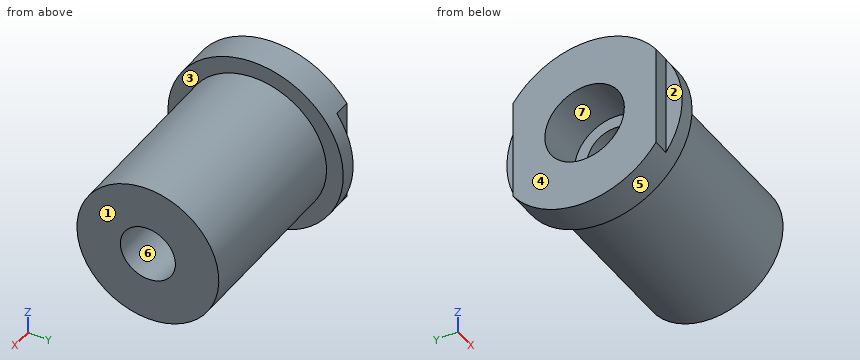
from build123d import *

# Parameters (mm, degrees)
ESQUISSE2_W                  = 103
ESQUISSE2_H                  = 43
ESQUISSE3_OUTSIDE_W          = 119.876
ESQUISSE3_OUTSIDE_H          = 119.876
ESQUISSE3_OUTSIDE_R          = 34.8
ENL_V_MAT_EXTRU_1_DEPTH      = 87
ENL_V_MAT_EXTRU_2_DEPTH      = 120.61187232
ENL_V_MAT_EXTRU_2_DEPTH_BACK = 8
ENL_V_MAT_EXTRU_3_DEPTH      = 120.61187232
ENL_V_MAT_EXTRU_3_DEPTH_BACK = 8
ESQUISSE7_R                  = 19.5
ENL_V_MAT_EXTRU_4_DEPTH      = 24
ESQUISSE8_R                  = 13.5
ENL_V_MAT_EXTRU_5_DEPTH      = 100.694533451


with BuildPart() as part:
    # Esquisse2 → Révolution1 (revolve)
    with BuildSketch(Plane.XY, mode=Mode.PRIVATE) as r_volution1_sk:
        with Locations((51.5, 21.5)):
            Rectangle(ESQUISSE2_W, ESQUISSE2_H)
    revolve(r_volution1_sk.sketch.rotate(Axis((103, 0, 0), (-1, 0, 0)), 90), axis=Axis((103, 0, 0), (-1, 0, 0)))

    # Esquisse3 outside → Enlèv. mat.-Extru.1 (cut)
    with BuildSketch(Plane(origin=(103, 0, 0), x_dir=(0, 0, -1), z_dir=(1, 0, 0))):
        Rectangle(ESQUISSE3_OUTSIDE_W, ESQUISSE3_OUTSIDE_H)
        Circle(ESQUISSE3_OUTSIDE_R, mode=Mode.SUBTRACT)
    extrude(amount=-ENL_V_MAT_EXTRU_1_DEPTH, mode=Mode.SUBTRACT)

    # Esquisse4 → Enlèv. mat.-Extru.2 (cut, two sides: drawn at the far end of the back side and taken through both)
    with BuildSketch(Plane.ZY.offset(-ENL_V_MAT_EXTRU_2_DEPTH_BACK)):
        Polygon((-241.912631386, 35), (-24.979991994, 35), (24.979991994, 35), (241.912631386, 35), (241.912631386, 468.865278784), (-241.912631386, 468.865278784), align=None)
    extrude(amount=ENL_V_MAT_EXTRU_2_DEPTH + ENL_V_MAT_EXTRU_2_DEPTH_BACK, mode=Mode.SUBTRACT)

    # Esquisse5 → Enlèv. mat.-Extru.3 (cut, two sides: drawn at the far end of the back side and taken through both)
    with BuildSketch(Plane.ZY.offset(-ENL_V_MAT_EXTRU_3_DEPTH_BACK)):
        Polygon((-241.912631386, -35), (-24.979991994, -35), (24.979991994, -35), (241.912631386, -35), (241.912631386, -468.865278784), (-241.912631386, -468.865278784), align=None)
    extrude(amount=ENL_V_MAT_EXTRU_3_DEPTH + ENL_V_MAT_EXTRU_3_DEPTH_BACK, mode=Mode.SUBTRACT)

    # Esquisse7 → Enlèv. mat.-Extru.4 (cut)
    with BuildSketch(Plane.ZY):
        Circle(ESQUISSE7_R)
    extrude(amount=-ENL_V_MAT_EXTRU_4_DEPTH, mode=Mode.SUBTRACT)

    # Esquisse8 → Enlèv. mat.-Extru.5 (cut, through all)
    with BuildSketch(Plane.ZY.offset(-24)):
        Circle(ESQUISSE8_R)
    extrude(amount=-ENL_V_MAT_EXTRU_5_DEPTH, mode=Mode.SUBTRACT)


solid = part.part
Input: part model. Units: mm. Frame: model coordinates. Face numbers are marked on the shaded views. A direction names the side the tool comes from. Coordinates: 2 decimals unless noted, no trailing zeros. Loops run counter-clockwise (first coordinate to the right, second up) from the corner with the lowest first, then second, coordinate; pieces in that order, holes last.
Q1. Cut plane A-A (y = 0). Output: boundary loops of the cut face in (x, z).
Q2. Contact query for flat-ended pins moving along their axis: pin 1 (6.5 mm diameter, centred on x = 2.5, z = 3.5, fed in from -Y); pin 2 (3 mm diameter, centred on x = 41, y = -15.5, fed in from -Z); pin 3 (5 mm diameter, centred on x = 14.5, z = -3, fed in from -Y); pin 4 (16 mm diameter, centred on y = 0, z = 0, fed in from -X). Output: stop coordinate, or through.
Q3. Draft query along Y for the marked faces 4, 5, 6 and 7. Return one class per face: +Y half, -Y half, draft (parallel to the pull), parting line (faces both ways), or undercut.
Q4. Material intervals for line 1 (Y direction, x = 5.5, z = 0); line 2 (Y direction, x = 11.25, z = 0); line 3 (X direction, y = 23.5, z = 27), sorted ascending.
Q5. Cut plane B-B (z = 0). Output: boundary loops of the cut face in (x, y), then the cut area to 3 significant figures.
Q6. Cut plane C-C (x = 43.5). Output: boundary loops of the cut face in (y, z).
Q7. Set-up query: the marked faces 1, 2 and 3. Return all of +Z, -Z, +X, -X, +Y, -Y with unobstructed straight access to the full face (end or side cutting, diameter ignored); none if empty.
Q8. Cut plane D-D (y = -22.5). Output: boundary loops of the cut face in (x, z), then the cut area to 3 significant figures.
Working result:
1. outline: (0, -43) - (16, -43) - (16, -34.8) - (103, -34.8) - (103, -13.5) - (24, -13.5) - (24, -19.5) - (0, -19.5) - close; (0, 19.5) - (24, 19.5) - (24, 13.5) - (103, 13.5) - (103, 34.8) - (16, 34.8) - (16, 43) - (0, 43) - close
2. pin 1: stops at y = -35
2. pin 2: stops at z = -31.86
2. pin 3: stops at y = -43
2. pin 4: passes through
3. face 4: draft
3. face 5: parting line
3. face 6: undercut
3. face 7: undercut
4. line 1: y = -35 to -19.5, 19.5 to 35
4. line 2: y = -43 to -19.5, 19.5 to 43
4. line 3: x = 0 to 16
5. outline: (0, -35) - (8, -35) - (8, -43) - (16, -43) - (16, -34.8) - (103, -34.8) - (103, -13.5) - (24, -13.5) - (24, -19.5) - (0, -19.5) - close; (0, 19.5) - (24, 19.5) - (24, 13.5) - (103, 13.5) - (103, 34.8) - (16, 34.8) - (16, 43) - (8, 43) - (8, 35) - (0, 35) - close
5. area: 4,230 mm2
6. outline: circle Ø69.6 at (0, 0); hole circle Ø27 at (0, 0)
7. face 1: +Z, -Z, +X, +Y, -Y
7. face 2: +Z, -Z, -X, -Y
7. face 3: +X
8. outline: (0, -36.64) - (16, -36.64) - (16, -26.55) - (103, -26.55) - (103, 26.55) - (16, 26.55) - (16, 36.64) - (0, 36.64) - close
8. area: 5,790 mm2
